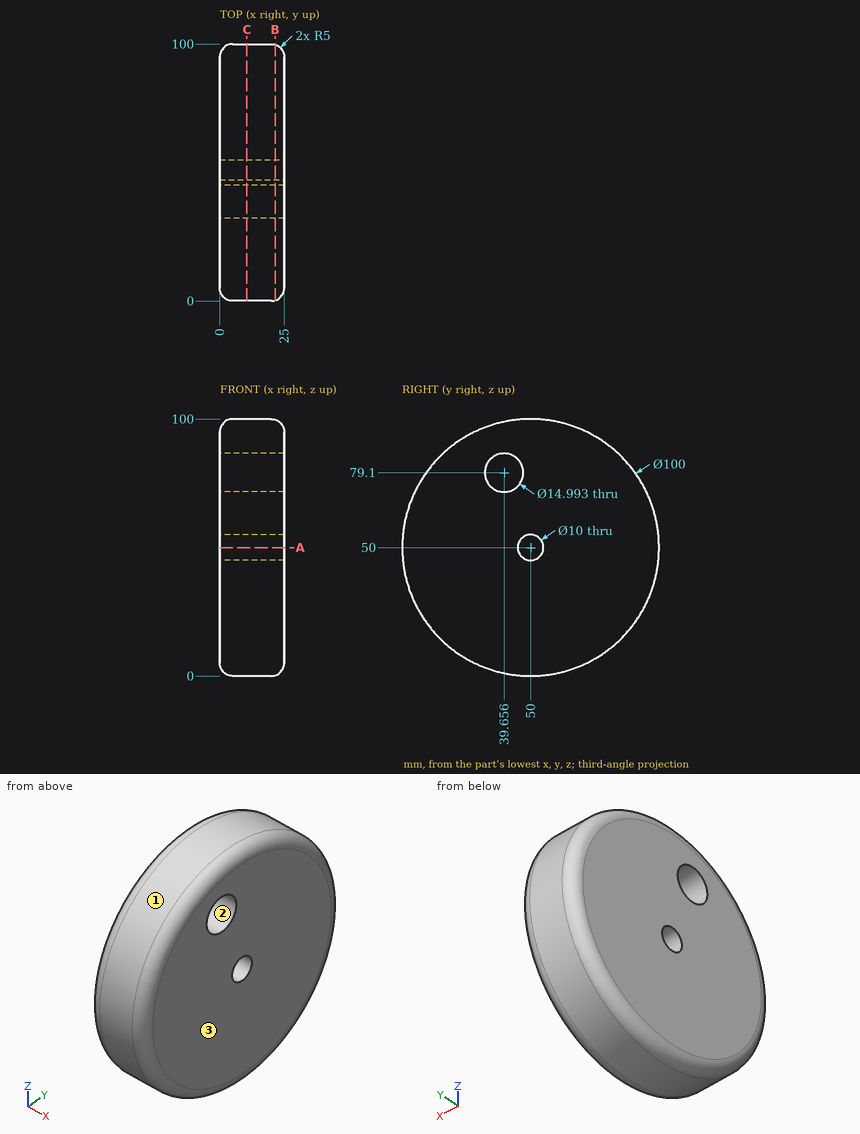
Job drawing, mm, ordinate dimensions from the low corner. One solid piece. Round coordinates to 2 decimals unless told otherwise and drop trailing zeros. Loops run counter-clockwise (first coordinate to the right, second up) from the corner with the lowest first, then second, coordinate; pieces in that order, holes last. Notation, with made-up numbers: M 70,55.25 L 82,55.25 A18 ccw 82,66.25 Z; hole C -4,-24 d3. An arc over 180 degrees is marked long. One line per question, with ' | ' between items. Start each with the question number.
Item 1: Cut at B-B, the plane x = 21.5. Write the cut outline in (y, z) (1 decimal).
Item 2: Cut at A-A, the plane z = 50. Write the cut outline in (x, y), plus the area to 3 significant figures.
Item 3: Wall check: line 1 (Z direction, x = 18.5, y = 50); line 2 (Z direction, x = 4, y = 36) (1 decimal); line 3 (Z direction, x = 3, y = 60) (1 decimal). Give the ranges that are in metal, low to high.
Item 4: Cut at C-C, the plane x = 10.5. Write the cut outline in (y, z) (1 decimal), plus the area to 3 significant figures.
Item 5: Pin check, flat tips, straight feed: pin 1 Ø8 at (x, y) = (5.5, 30.5) entering from -Z; pin 2 Ø1 at (x, y) = (15.5, 30.5) entering from +Z; pin 3 Ø1 at (x, z) = (10, 25) entering from -Y; pin 4 Ø9 at (y, z) = (39.66, 79.1) entering from +X. Stop position of each tip, or through.
Item 6: Two-plate mould, pull along Z, no slides. Class the marked faces 1, 2 and 3: pulls with the +Z half, pulls with the -Z half, needs draft (parallel to the pull), parting line crosses it, or undercut.
Responses:
1) outline: C 50,50 d99.5; hole C 39.7,79.1 d15; hole C 50,50 d10
2) outline: M 0,5 A5 ccw 5,0 L 20,0 A5 ccw 25,5 L 25,45 L 0,45 Z; M 0,55 L 25,55 L 25,95 A5 ccw 20,100 L 5,100 A5 ccw 0,95 Z | area: 2,230 mm²
3) line 1: z = 0 to 45, 55 to 100 | line 2: z = 2.1 to 72.6, 85.6 to 97.9 | line 3: z = 1.4 to 98.6
4) outline: C 50,50 d100; hole C 39.7,79.1 d15; hole C 50,50 d10 | area: 7,600 mm²
5) pin 1: stops at z = 2.46 | pin 2: stops at z = 96.25 | pin 3: stops at y = 6.41 | pin 4: passes through
6) face 1: parting line crosses it | face 2: undercut | face 3: needs draft
